Can you work these out from the model? Positions are in its coordinate system, mm. Face numbers are marked on the shaded views. Give positions to 0.01 mm unless a question says otherwise; leave off trailing zeros. Loops run counter-clockwise (first coordinate to the right, second up) from the corner with the lowest first, then second, coordinate; pieces in that order, holes last. Notation, with made-up numbers: M 77.25,12.25 L 107.25,12.25 A22 ccw 107.25,21.25 Z; hole C -12.75,27 d6. An arc over 180 degrees is marked long. One line per item, written item: value. Start each with the question number.
Autodesk Inventor part; units mm, degrees
ref_plane "YZ Plane" through (0, 0, 0) normal (1, 0, 0) x (0, 1, 0)
ref_plane "XZ Plane" through (0, 0, 0) normal (0, 1, 0) x (-1, 0, 0)
ref_plane "XY Plane" through (0, 0, 0) normal (0, 0, 1) x (1, 0, 0)
sketch "CONTOURS" plane through (0, 0, 0) normal (0, 0, 1) x (1, 0, 0)
  arc A0 (1567.8979, 1059.3694) -> (1592.5572, 1062.5103) centre (1579.0574, 1070.1265) ccw
  line L0 (1592.5572, 1062.5103) -> (1600.8567, 1077.2212)
  arc A1 (1623.3344, 1080.7382) -> (1600.8567, 1077.2212) centre (1613.4855, 1070.0964) ccw
  line L1 (1623.3344, 1080.7382) -> (1755.4047, 958.5078)
  arc A2 (1752.9302, 935.3813) -> (1755.4047, 958.5078) centre (1745.5558, 947.866) ccw
  line L2 (1752.9302, 935.3813) -> (1728.0763, 920.7006)
  arc A3 (1728.0763, 920.7006) -> (1724.7998, 896.5978) centre (1735.9593, 907.3549) ccw
  line L3 (1724.7998, 896.5978) -> (1764.2337, 855.6886)
  arc A4 (25.6661, 904.4304) -> (1764.2337, 855.6886) centre (918.8737, 1733.3946) ccw
  line L4 (25.6661, 904.4304) -> (308.0876, 1099.0382)
  arc A5 (308.0876, 1099.0382) -> (1529.6596, 1099.0382) centre (918.8736, 1733.3944) ccw
  line L5 (1529.6596, 1099.0382) -> (1567.8979, 1059.3694)
  dimension "d1" = 1218.6064
  dimension "d3" = 880.6062
sketch "HOLES" plane through (0, 0, 0) normal (0, 0, 1) x (1, 0, 0)
  line L0 (376.9652, 673.5139) -> (381.8614, 683.3642)
  arc A0 (387.2238, 685.1656) -> (381.8614, 683.3642) centre (385.4433, 681.5837) ccw
  line L1 (387.2238, 685.1656) -> (419.4609, 669.1416)
  arc A1 (421.2623, 663.7792) -> (419.4609, 669.1416) centre (417.6804, 665.5597) ccw
  arc A2 (1631.4879, 1048.1109) -> (1625.8313, 1048.0547) centre (1628.6877, 1045.2545) ccw
  line L2 (1718.6644, 957.049) -> (1710.9639, 949.1939)
  arc A3 (1705.3073, 949.1377) -> (1710.9639, 949.1939) centre (1708.1075, 951.9941) ccw
  line L3 (1705.3073, 949.1377) -> (1618.1871, 1034.543)
  arc A4 (1618.1309, 1040.1996) -> (1618.1871, 1034.543) centre (1620.9873, 1037.3994) ccw
  line L4 (1618.1309, 1040.1996) -> (1625.8313, 1048.0547)
  line L5 (1631.4879, 1048.1109) -> (1718.6081, 962.7056)
  arc A5 (1718.6644, 957.049) -> (1718.6081, 962.7056) centre (1715.808, 959.8492) ccw
  line L6 (497.3235, 915.6504) -> (502.2197, 925.5006)
  arc A6 (507.5821, 927.3021) -> (502.2197, 925.5006) centre (505.8016, 923.7202) ccw
  line L7 (507.5821, 927.3021) -> (539.8192, 911.2781)
  arc A7 (541.6206, 905.9157) -> (539.8192, 911.2781) centre (538.0387, 907.6962) ccw
  line L8 (416.4201, 741.8384) -> (470.5996, 851.148)
  arc A8 (531.362, 894.264) -> (536.7244, 896.0655) centre (533.1425, 897.8459) ccw
  line L9 (531.362, 894.264) -> (499.1249, 910.2881)
  arc A9 (497.3235, 915.6504) -> (499.1249, 910.2881) centre (500.9054, 913.87) ccw
  line L10 (479.5438, 851.1791) -> (485.8157, 848.0705)
  arc A10 (487.6232, 842.7102) -> (485.8157, 848.0705) centre (484.0393, 844.4865) ccw
  line L11 (487.6232, 842.7102) -> (433.4437, 733.4006)
  arc A11 (428.0834, 731.5931) -> (433.4437, 733.4006) centre (429.8598, 735.177) ccw
  line L12 (428.0834, 731.5931) -> (418.2276, 736.4781)
  arc A12 (416.4201, 741.8384) -> (418.2276, 736.4781) centre (420.004, 740.062) ccw
  line L13 (541.6206, 905.9157) -> (536.7244, 896.0655)
  arc A13 (475.9599, 852.9555) -> (470.5996, 851.148) centre (474.1835, 849.3716) ccw
  line L14 (475.9599, 852.9555) -> (479.5438, 851.1791)
  line L15 (421.2623, 663.7792) -> (416.3661, 653.929)
  arc A14 (411.0038, 652.1276) -> (416.3661, 653.929) centre (412.7842, 655.7095) ccw
  line L16 (411.0038, 652.1276) -> (378.7667, 668.1516)
  arc A15 (376.9652, 673.5139) -> (378.7667, 668.1516) centre (380.5471, 671.7335) ccw
  dimension "d5" = 0.065
  dimension "d7" = 0.065
sketch "LETTERS" plane through (0, 0, 0) normal (0, 0, 1) x (1, 0, 0)
  line L0 (544.6299, 751.705) -> (554.564, 747.8187)
  line L1 (561.8694, 755.3769) -> (548.1913, 760.7277)
  line L2 (548.1913, 760.7277) -> (540.975, 742.2812)
  line L3 (540.975, 742.2812) -> (554.6531, 736.9303)
extrude "Extrusion3" add sketch "CONTOURS" along normal blind 18
extrude "Extrusion4" cut sketch "HOLES" along normal blind 18
properties part number "Platform E1" material "Wood (Birch)"
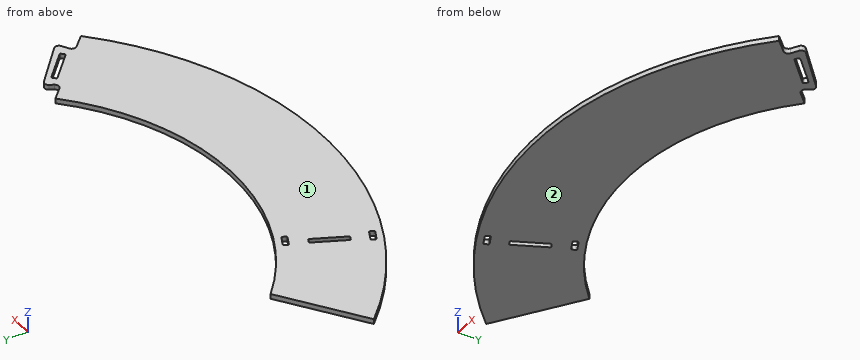
Q1. If we section it at D-D, the plane x = 201: Write out the boundary of the cut face in (y, z), plus the area to 3 significant figures.
Q2. I need wall thicknesses on line 1 along X through (y, z) = (980, 14.5); line 2 along X through (y, z) = (925.5, 5); line 3 along X through (y, z) = (795.5, 2.75). Which ranges of each line are inside material? Lowest first, please.
Q3. If we section it at B-B, the plane y = 802: Write out the boundary of the cut face in (x, z), plus the area to 3 significant figures.
Q4. If we section it at C-C, the plane z = 7: Give the number of separate pieces and of enclosed holes in the cut face, plus the area to 3 significant figures.
Q5. If we mould it in two halves opening along Z, with no side actions, what happens to the marked faces 1 and 2? For each: released by +Z, released by -Z, zero draft, split by the parting line, or undercut.
Q6. For P1, Ø5, axis at y = 635.5, z = 12.5, coming from the +X side; P2, Ø4, axis at y = 1001.5, z = 13.5, coming from the -X side; P3, Ø3, axis at y = 809.5, z = 9.5, coming from the +X side, each with a flat end and sliding along its axis, tell me the tip position at first contact or that it passes through.
Q7. If we section it at A-A, the plane y = 985: Write out the boundary of the cut face in (x, z).
Response:
1. outline: M 748.68,0 L 1025.25,0 L 1025.25,18 L 748.68,18 Z
1. area: 4,980 mm^2
2. line 1: 135.34 to 462.95, 1374.79 to 1673.83, 1700.97 to 1732.18
2. line 2: 56.24 to 502.22, 511.21 to 568.48, 1269.26 to 1736.2
2. line 3: 140.83 to 443.02, 464.22 to 1696.92
3. outline: M 133.06,0 L 446.24,0 L 446.24,18 L 133.06,18 Z; M 467.45,0 L 1704.69,0 L 1704.69,18 L 467.45,18 Z
3. area: 27,900 mm^2
4. separate pieces: 1
4. enclosed holes: 4
4. area: 561,000 mm^2
5. face 1: released by +Z
5. face 2: released by -Z
6. P1: x = 1452.83
6. P2: x = 163.63
6. P3: x = 1715.23
7. outline: M 142.59,0 L 454.79,0 L 454.79,18 L 142.59,18 Z; M 1382.96,0 L 1668.72,0 L 1668.72,18 L 1382.96,18 Z; M 1695.87,0 L 1726.78,0 L 1726.78,18 L 1695.87,18 Z
